Solid Edge part; units mm, degrees
sketch "Sketch1" plane through (0, 0, 0) normal (0, 0, 1) x (1, 0, 0)
  line L0 (-59.75, -14) -> (59.75, -14)
  line L1 (59.75, -14) -> (59.75, 14)
  line L2 (59.75, 14) -> (-59.75, 14)
  line L3 (-59.75, 14) -> (-59.75, -14)
extrude "Protrusion1" add sketch "Sketch1" against normal blind 40
sketch "Sketch2" plane through (0, -14, -20) normal (0, -1, 0) x (1, 0, 0)
  line L0 (-59.75, 20) -> (-41.25, 20)
  line L1 (-41.25, 20) -> (-41.25, 8)
  line L2 (-41.25, 8) -> (-59.75, 8)
  line L3 (-59.75, 8) -> (-59.75, 20)
extrude "ExtrudedCutout_1" cut sketch "Sketch2" against normal blind 28
sketch "Sketch3" plane through (0, -14, -20) normal (0, -1, 0) x (1, 0, 0)
  line L0 (59.75, 20) -> (41.25, 20)
  line L1 (41.25, 20) -> (41.25, 8)
  line L2 (41.25, 8) -> (59.75, 8)
  line L3 (59.75, 8) -> (59.75, 20)
extrude "ExtrudedCutout_2" cut sketch "Sketch3" against normal blind 28
sketch "Sketch4" plane through (0, -14, -20) normal (0, -1, 0) x (1, 0, 0)
  line L0 (41.25, 20) -> (35.75, 20)
  line L1 (35.75, 20) -> (41.25, 8)
  line L2 (41.25, 8) -> (41.25, 20)
extrude "ExtrudedCutout_3" cut sketch "Sketch4" against normal blind 28
sketch "Sketch5" plane through (0, -14, -20) normal (0, -1, 0) x (1, 0, 0)
  line L0 (-41.25, 20) -> (-35.75, 20)
  line L1 (-35.75, 20) -> (-41.25, 8)
  line L2 (-41.25, 8) -> (-41.25, 20)
extrude "ExtrudedCutout_4" cut sketch "Sketch5" against normal blind 28
sketch "Sketch6" plane through (59.75, 0, -26) normal (1, 0, 0) x (0, 1, 0)
  line L0 (-4.65, 26) -> (-4.65, -8)
  line L1 (-4.65, -8) -> (4.65, -8)
  line L2 (4.65, -8) -> (4.65, 26)
  line L3 (4.65, 26) -> (-4.65, 26)
extrude "ExtrudedCutout_5" cut sketch "Sketch6" against normal blind 119.5
chamfer "Chamfer_1" distance 6 angle 45 1 edges at (0, 4.65, 0)
chamfer "Chamfer_2" distance 6 angle 45 1 edges at (0, -4.65, 0)
sketch "Sketch7" plane through (50.5, 9.325, -12) normal (0, 0, 1) x (0, 1, 0)
  line L0 (-4.675, -9.25) -> (-2.675, -9.25)
  line L1 (-2.675, -9.25) -> (-4.675, 9.25)
  line L2 (-4.675, 9.25) -> (-4.675, -9.25)
extrude "ExtrudedCutout_6" cut sketch "Sketch7" against normal blind 22
sketch "Sketch8" plane through (50.5, -9.325, -12) normal (0, 0, 1) x (0, 1, 0)
  line L0 (4.675, -9.25) -> (2.675, -9.25)
  line L1 (2.675, -9.25) -> (4.675, 9.25)
  line L2 (4.675, 9.25) -> (4.675, -9.25)
extrude "ExtrudedCutout_7" cut sketch "Sketch8" against normal blind 22
sketch "Sketch9" plane through (-50.5, -9.325, -12) normal (0, 0, 1) x (0, 1, 0)
  line L0 (4.675, 9.25) -> (2.675, 9.25)
  line L1 (2.675, 9.25) -> (4.675, -9.25)
  line L2 (4.675, -9.25) -> (4.675, 9.25)
extrude "ExtrudedCutout_8" cut sketch "Sketch9" against normal blind 22
sketch "Sketch10" plane through (-50.5, 9.325, -12) normal (0, 0, 1) x (0, 1, 0)
  line L0 (-4.675, 9.25) -> (-2.675, 9.25)
  line L1 (-2.675, 9.25) -> (-4.675, -9.25)
  line L2 (-4.675, -9.25) -> (-4.675, 9.25)
extrude "ExtrudedCutout_9" cut sketch "Sketch10" against normal blind 22
chamfer "Chamfer_5" distance 18.5 distance2 2 1 edges at (59.75, 0, -34) measured on face at (-38.6383, -4.5663, -34)
chamfer "Chamfer_6" distance 18.5 distance2 2 1 edges at (-59.75, 0, -34) measured on face at (-41.9067, -4.5663, -34)
Source: CAD feature listing. Evaluate the final solid. Frame: model axes, mm. A direction names the side the tool comes from. Give positions to 0.01 mm unless a question says otherwise; leave off trailing zeros. Loops run counter-clockwise (first coordinate to the right, second up) from the corner with the lowest first, then second, coordinate; pieces in that order, holes last. Notation, with made-up numbers: (-17, 62) -> (17, 62) arc R12 ccw to (17, 74) -> close; hole circle Ø9 at (41, -19.75). An arc over 180 degrees is marked (long way). Use a Markdown table: item, result. Add a question column.
(1) Section query C-C (x = -11.5). Output: boundary loops of the cut face in (y, z), then the cut area to 3 significant figures.
(2) Section query A-A (z = -29.5). Output: boundary loops of the cut face in (x, y).
(3) Ray query, line 1 (Y direction, x = -3.5, z = -23); line 2 (Z direction, x = -52.5, y = -9.25); line 3 (Z direction, x = 25, y = 3.75). Return the intervals inside material, ascending.
(4) First-contact query: pin 1 Ø4.5 at (x, y) = (-14, -0.5) entering from +Z; pin 2 Ø3 at (x, y) = (-47, 11.5) entering from +Z; pin 3 Ø2 at (x, y) = (12, 7.5) entering from +Z. Flat tips, straight axial feed; report the tip coordinate or a pass-through.
(5) Section query D-D (z = -4.5). Output: boundary loops of the cut face in (x, y), then the cut area to 3 significant figures.
(6) Section query B-B (y = 8.25). Output: boundary loops of the cut face in (x, z).
(7) Pull-direction query (Y, two-part tool) for faces 5 (the face through (-1, -14, -20)), 6 (the face through (1, 0, -34)), 7 (the face through (50, 9, -12)); classes: +Y half, -Y half, draft (parallel to the pull), parting line (faces both ways), or undercut.
(8) Access query for faces 1 (the face through (0.54, 7.69, -2.96)), 2 (the face through (50, -9, -12)), 3 (the face through (-50.63, 0.093, -35.014)), 4 (the face through (-50, 9, -12)). Directions: +Z, -Z, +X, -X, +Y, -Y. A direction counts if a zero-diameter tool reaches every point of the face in a straight line with its end or side. Return the directions, or none.
Checked values:
| question | item | result |
|---|---|---|
| 1 | outline | (-14, -40) -> (14, -40) -> (14, 0) -> (10.65, 0) -> (4.65, -6) -> (4.65, -34) -> (-4.65, -34) -> (-4.65, -6) -> (-10.65, 0) -> (-14, 0) -> close |
| 1 | area | 768 mm^2 |
| 2 | outline | (-59.75, -14) -> (59.75, -14) -> (59.75, -6.65) -> (41.25, -4.65) -> (-41.25, -4.65) -> (-59.75, -6.65) -> close; (-59.75, 6.65) -> (-41.25, 4.65) -> (41.25, 4.65) -> (59.75, 6.65) -> (59.75, 14) -> (-59.75, 14) -> close |
| 3 | line 1 | -14 to -4.65, 4.65 to 14 |
| 3 | line 2 | -40 to -12 |
| 3 | line 3 | -40 to -34 |
| 4 | pin 1 | z = -34 |
| 4 | pin 2 | z = -12 |
| 4 | pin 3 | z = -2.15 |
| 5 | outline | (-37.81, -14) -> (37.81, -14) -> (37.81, -6.15) -> (-37.81, -6.15) -> close; (-37.81, 6.15) -> (37.81, 6.15) -> (37.81, 14) -> (-37.81, 14) -> close |
| 5 | area | 1,190 mm^2 |
| 6 | outline | (-59.75, -40) -> (59.75, -40) -> (59.75, -12) -> (41.25, -12) -> (36.85, -2.4) -> (-36.85, -2.4) -> (-41.25, -12) -> (-59.75, -12) -> close |
| 7 | face 5 | -Y half |
| 7 | face 6 | undercut |
| 7 | face 7 | draft |
| 8 | face 1 | +Z, +X, -X |
| 8 | face 2 | +Z, +X, +Y, -Y |
| 8 | face 3 | +Z, -X |
| 8 | face 4 | +Z, -X, +Y, -Y |
